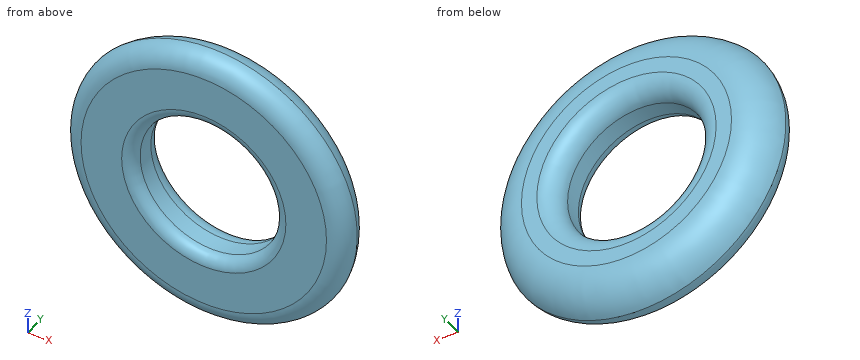
from build123d import *

# Parameters (mm, degrees)
F0_R     = 9.525
F0_R_2   = 4.7625
F1_DEPTH = 3.175
F2_R     = 1.27
F4_R     = 1.27
F5_R     = 0.762


# Not quite as in the source:
# - a fillet or chamfer that OpenCascade refuses, or shapes differently, is made with other operations: its cross-section is extruded or revolved along the edge and cut away or added


with BuildPart() as f1:
    # F0 (on Front) → F1 (new body)
    with BuildSketch(Plane.XZ):
        Circle(F0_R)
        Circle(F0_R_2, mode=Mode.SUBTRACT)
    extrude(amount=F1_DEPTH)

    # F2
    f2_edges = [f1.edges().sort_by_distance(p)[0] for p in [
        (-9.525, -3.175, 0),
    ]]
    fillet(f2_edges, radius=F2_R)

    # F3: fillet of radius 2.54 on 1 edges, made by hand

    # F3_s1 → F3_t2 (revolve, cut)
    with BuildSketch(Plane.XY):
        with BuildLine():
            ThreePointArc((9.525, -1.905), (8.6210815618, -0.5319536858), (7.0656555752, 0))
            Line((7.0656555752, 0), (7.0656555752, 0.0508))
            Line((7.0656555752, 0.0508), (9.525, 0.0508))
            Line((9.525, 0.0508), (9.5758, 0))
            ThreePointArc((9.5758, 0), (9.5758, -0.9525), (9.5741868885, -1.8923))
            Line((9.5741868885, -1.8923), (9.525, -1.905))
        make_face()
    revolve(axis=Axis((0, 0, 0), (0, -1, 0)), mode=Mode.SUBTRACT)

    # F4
    f4_edges = [f1.edges().sort_by_distance(p)[0] for p in [
        (-4.7625, 0, 0),
    ]]
    fillet(f4_edges, radius=F4_R)

    # F5
    f5_edges = [f1.edges().sort_by_distance(p)[0] for p in [
        (-4.7625, -3.175, 0),
    ]]
    fillet(f5_edges, radius=F5_R)


solid = f1.part
Geometry check sheet. Reference: the model listing, model coordinates, mm. Give positions to 0.01 mm unless a question says otherwise; leave off trailing zeros. Loops run counter-clockwise (first coordinate to the right, second up) from the corner with the lowest first, then second, coordinate; pieces in that order, holes last.
(1) Thickness scan on L1, parallel to Z at x = 0, y = -1.55; L2, parallel to X at y = -2.35, z = -3; L3, parallel to Z at x = 4.25, y = -1.9. Record the ranges inside material, lowest first.
From the geometry:
L1: z = -9.4 to -4.76, 4.76 to 9.4
L2: x = -8.96 to -3.7, 3.7 to 8.96
L3: z = -8.52 to -2.15, 2.15 to 8.52
(2) Depth check by flat-ended pin: pin 1 Ø1.5 at (x, y) = (-2, -1.5) entering from -Z; pin 2 Ø1.5 at (y, z) = (-2, -4.5) entering from -X; pin 3 Ø1 at (y, z) = (-1.5, 6) entering from -X. Enter the tip coordinate at first touch or a pass-through.
From the geometry:
pin 1: stops at z = -9.43
pin 2: stops at x = -8.75
pin 3: stops at x = -7.67
(3) Section check D-D on y = -1.55. Record the cut outline in (x, z) (1 decimal), then the cut area to 3 significant figures.
From the geometry:
outline: circle Ø18.8 at (0, 0); hole circle Ø9.5 at (0, 0)
area: 207 mm2
(4) Section check A-A on x = 0. Record the cut outline in (y, z) (1 decimal).
From the geometry:
outline: (-3.2, -8.3) arc R1.3 ccw to (-1.9, -9.5) arc R2.5 ccw to (0, -7.1) - (0, -6) arc R1.3 ccw to (-1.3, -4.8) - (-2.4, -4.8) arc R0.8 ccw to (-3.2, -5.5) - close; (-3.2, 5.5) arc R0.8 ccw to (-2.4, 4.8) - (-1.3, 4.8) arc R1.3 ccw to (0, 6) - (0, 7.1) arc R2.5 ccw to (-1.9, 9.5) arc R1.3 ccw to (-3.2, 8.3) - close
(5) Section check B-B on z = 0. Record the cut outline in (x, y) (1 decimal), then the cut area to 3 significant figures.
From the geometry:
outline: (-9.5, -1.9) arc R1.3 ccw to (-8.3, -3.2) - (-5.5, -3.2) arc R0.8 ccw to (-4.8, -2.4) - (-4.8, -1.3) arc R1.3 ccw to (-6, 0) - (-7.1, 0) arc R2.5 ccw to start; (4.8, -2.4) arc R0.8 ccw to (5.5, -3.2) - (8.3, -3.2) arc R1.3 ccw to (9.5, -1.9) arc R2.5 ccw to (7.1, 0) - (6, 0) arc R1.3 ccw to (4.8, -1.3) - close
area: 26.2 mm2
(6) Section check C-C on y = -0.25. Record the cut outline in (x, z).
From the geometry:
outline: circle Ø16.33 at (0, 0); hole circle Ø10.55 at (0, 0)
